```python
from build123d import *

# Parameters (mm, degrees)
F1_W      = 36.2
F1_H      = 38.8
F2_W      = 12.866667
F2_H      = 38.8
F3_FACE_W = 36.2
F3_FACE_H = 38.8
F4_DEPTH  = 12
F5_W      = 13.8
F5_H      = 13.8
F6_DEPTH  = 31
F7_W      = 20
F7_H      = 22.8
F8_DEPTH  = 3.2
F9_W      = 14
F9_H      = 9.3
F10_DEPTH = 31


with BuildPart() as f3:
    # F1 (on offset) → F3 section 0
    with BuildSketch(Plane.XY.offset(36.125)):
        with Locations((0, -19.4)):
            Rectangle(F1_W, F1_H)
    # F2 (on Top) → F3 section 1
    with BuildSketch(Plane.XY):
        with Locations((-3.3e-05, -19.4)):
            Rectangle(F2_W, F2_H)
    loft()

    # F3_face (on face) → F4 (cut)
    with BuildSketch(Plane(origin=(0, -19.4, 36.125), x_dir=(1, 0, 0), z_dir=(0, 0, 1))):
        Rectangle(F3_FACE_W, F3_FACE_H)
    extrude(amount=-F4_DEPTH, mode=Mode.SUBTRACT)

    # F5 (on offset) → F6 (cut)
    with BuildSketch(Plane.XY.offset(36.125)):
        with Locations((0, -19.4)):
            Rectangle(F5_W, F5_H)
    extrude(amount=-F6_DEPTH, mode=Mode.SUBTRACT)

    # F7 (on Top) → F8 (cut)
    with BuildSketch(Plane.XY):
        with Locations((0, -19.4)):
            Rectangle(F7_W, F7_H)
    extrude(amount=F8_DEPTH, mode=Mode.SUBTRACT)

    # F9 (on offset) → F10 (cut)
    with BuildSketch(Plane.XY.offset(36.125)):
        with Locations((0, -6.25)):
            Rectangle(F9_W, F9_H)
        with Locations((0, -32.55)):
            Rectangle(F9_W, F9_H)
    extrude(amount=-F10_DEPTH, mode=Mode.SUBTRACT)


solid = f3.part
```
Verification items for the finished model (mm, model axes). A direction names the side the tool comes from. Give positions to 0.01 mm unless a question says otherwise; leave off trailing zeros. Loops run counter-clockwise (first coordinate to the right, second up) from the corner with the lowest first, then second, coordinate; pieces in that order, holes last.
1. Go/stop test with flat-tipped pins: pin 1 Ø4 at (y, z) = (-18, 13) entering from +X; pin 2 Ø6 at (y, z) = (-27.5, 3.5) entering from -X; pin 3 Ø3 at (y, z) = (-34, 18.5) entering from -X. Record where each tip stops, or that it passes through.
2. Set-up check for faces 1 (the flat face through (0, -32, 5.125)), 2 (the flat face through (0, -8, 2)), 3 (the flat face through (9, -19, 24.125)): record each of +Z, -Z, +X, -X, +Y, -Y from which the full face is reachable in a straight line by a thin tool's end or side.
3. Section check A-A, the plane y = -33. Enter the section's corners in (x, z) (3 decimals), then the cut area to 3 significant figures.
4. Section check C-C, the plane z = 21.75. Count the separate pieces of the cut face and the enclosed holes in it, then the cut area to 3 significant figures.
5. Section check B-B, the plane y = -16. Enter the section's corners in (x, z) (3 decimals).
6. Thickness scan on line 1 (Y direction, x = -4.5, z = 12.25); line 2 (Z direction, x = -5.5, y = -23) (3 decimals); line 3 (X direction, y = -36, z = 5.25). Record the ranges inside material, lowest first.
7. Mould release check, pull along X, two halves, no side actions. Record for faces 4 (the flat face through (0, -30.8, 2)), 5 (the flat face through (10.274, -19.672, 11.894)), 6 (the flat face through (0, -6, 5.125)): released by +X, released by -X, zero draft, split by the parting line, or undercut.
Geometry says:
1. pin 1: stops at x = 11.28
1. pin 2: stops at x = -8.53
1. pin 3: stops at x = -12.89
2. face 1: +Z
2. face 2: -Z, +X, -X
2. face 3: +Z, +X, -X, +Y, -Y
3. outline: (-14.225, 24.125) - (-6.433, 0) - (6.433, 0) - (14.225, 24.125) - (7, 24.125) - (7, 5.125) - (-7, 5.125) - (-7, 24.125) - close
3. area: 232 mm2
4. separate pieces: 1
4. enclosed holes: 3
4. area: 593 mm2
5. outline: (-14.225, 24.125) - (-7.467, 3.2) - (7.467, 3.2) - (14.225, 24.125) - (6.9, 24.125) - (6.9, 5.125) - (-6.9, 5.125) - (-6.9, 24.125) - close
6. line 1: y = -38.8 to -37.2, -27.9 to -26.3, -12.5 to -10.9, -1.6 to 0
6. line 2: z = 3.2 to 5.125
6. line 3: x = -8.13 to -7, 7 to 8.13
7. face 4: zero draft
7. face 5: released by +X
7. face 6: undercut
